CAD build for the part. Positions are in the model's coordinates, mm. A direction names the side the tool comes from. Round coordinates to 2 decimals unless told otherwise and drop trailing zeros. Order: outer loops, then holes, each group sorted by start corner. A loop starts at its lowest first (then second) coordinate and runs counter-clockwise, first axis right, second up.
```python
from build123d import *

# Parameters (mm, degrees)
EXTRUDE_2_DEPTH          = 12.2
SKETCH_5_W               = 3
SKETCH_5_H               = 8.5
CUT_EXTRUDE_1_DEPTH      = 22.5
SKETCH_6_R               = 1.4
EXTRUDE_3_DEPTH          = 2.5
SKETCH_7_W               = 12.2
SKETCH_7_H               = 1
CUT_EXTRUDE_2_DEPTH      = 1
CUT_EXTRUDE_2_DEPTH_BACK = 32.1
EXTRUDE_4_DEPTH          = 0.2
EXTRUDE_5_DEPTH          = 0.2
SKETCH_10_W              = 32.1
SKETCH_10_H              = 20.5
EXTRUDE_6_DEPTH          = 2
SKETCH_11_W              = 32.1
SKETCH_11_H              = 20.5
EXTRUDE_7_DEPTH          = 2


with BuildPart() as part:
    # 草图4 → 凸台-拉伸2 (new body)
    with BuildSketch(Plane.XY):
        Polygon((-11.55, 0), (11.55, 0), (11.55, 17), (16.05, 17), (16.05, -4.5), (-16.05, -4.5), (-16.05, 17), (-11.55, 17), align=None)
    extrude(amount=EXTRUDE_2_DEPTH)

    # 草图5 → 切除-拉伸1 (cut, through all)
    with BuildSketch(Plane.XZ.offset(4.5)):
        with Locations((-10.05, 4.25)):
            Rectangle(SKETCH_5_W, SKETCH_5_H)
    extrude(amount=-CUT_EXTRUDE_1_DEPTH, mode=Mode.SUBTRACT)

    # 草图6 → 凸台-拉伸3 (add)
    with BuildSketch(Plane(origin=(0, 17, 0), x_dir=(1, 0, 0), z_dir=(0, 1, 0))):
        with Locations((13.8, -6.1)):
            Circle(SKETCH_6_R)
        with Locations((-13.8, -6.1)):
            Circle(SKETCH_6_R)
    extrude(amount=EXTRUDE_3_DEPTH)

    # 草图7 → 切除-拉伸2 (cut, two sides)
    with BuildSketch(Plane(origin=(16.05, 0, 0), x_dir=(0, 0, -1), z_dir=(1, 0, 0))) as cut_extrude_2_sk:
        with Locations((-6.1, -4)):
            Rectangle(SKETCH_7_W, SKETCH_7_H)
    extrude(amount=CUT_EXTRUDE_2_DEPTH, mode=Mode.SUBTRACT)
    extrude(cut_extrude_2_sk.sketch, amount=-CUT_EXTRUDE_2_DEPTH_BACK, mode=Mode.SUBTRACT)

    # 草图8 → 凸台-拉伸4 (add)
    with BuildSketch(Plane.XY.offset(12.2)):
        Polygon((-11.55, 17), (-16.05, 17), (-16.05, -3.5), (16.05, -3.5), (16.05, 17), (11.55, 17), (11.55, 0), (-11.55, 0), align=None)
    extrude(amount=EXTRUDE_4_DEPTH)

    # 草图9 → 凸台-拉伸5 (add)
    with BuildSketch(Plane.XY.offset(12.4)):
        Polygon((-11.55, 0), (-11.55, 17), (-16.05, 17), (-16.05, -3.5), (16.05, -3.5), (16.05, 17), (11.55, 17), (11.55, 0), align=None)
    extrude(amount=EXTRUDE_5_DEPTH)

    # 草图10 → 凸台-拉伸6 (add)
    with BuildSketch(Plane.XY.offset(12.6)):
        with Locations((0, 6.75)):
            Rectangle(SKETCH_10_W, SKETCH_10_H)
    extrude(amount=EXTRUDE_6_DEPTH)

    # 草图11 → 凸台-拉伸7 (add)
    with BuildSketch(Plane(origin=(0, 0, 0), x_dir=(-1, 0, 0), z_dir=(0, 0, -1))):
        with Locations((0, 6.75)):
            Rectangle(SKETCH_11_W, SKETCH_11_H)
    extrude(amount=EXTRUDE_7_DEPTH)


solid = part.part
```
1. Drill centre lines: line 1 (X direction, y = -0.75, z = 0.25); line 2 (Z direction, x = -9.5, y = 12); line 3 (X direction, y = 14, z = 2). Where is each one in solid material? Low to high.
2. Cut at B-B, the plane x = -9. Write the cut outline in (y, z).
3. Tool access for faces 5 (the face through (-8.55, -2, 4)), 6 (the face through (11.55, 9, 6)), 7 (the face through (0, 7, -2)): list every direction of +Z, -Z, +X, -X, +Y, -Y with a clear straight run to the whole face (end or side of a thin tool).
4. Mould opens along X. For faces 1 (the face through (14, 19.5, 6)), 2 (the face through (16.05, 7, 6)), 3 (the face through (-16.05, 7, 6)), 4 (the face through (-10, -2, 8.5)) say: released by +X, released by -X, zero draft, split by the parting line, or undercut.
5. Cut at C-C, the plane y = 10.75. Write the cut outline in (x, z), and give its area (3 significant figures).
6. Pin check, flat tips, straight feed: P1, Ø8.5, axis at x = 4.5, z = 4, coming from the +Y side; P2, Ø4, axis at x = 3, z = 4, coming from the +Y side. Stop position of each tip, or through.
7. Cut at A-A, the plane z = 6.1. Write the cut outline in (x, y).
8. Cut at D-D, the plane x = 9. Write the cut outline in (y, z), and give its area (3 significant figures).
Outcome:
1. line 1: x = -16.05 to -11.55, -8.55 to 16.05
1. line 2: z = -2 to 0, 12.6 to 14.6
1. line 3: x = -16.05 to -11.55, 11.55 to 16.05
2. outline: (-3.5, -2) - (17, -2) - (17, 0) - (-3.5, 0) - close; (-3.5, 8.5) - (0, 8.5) - (0, 12.6) - (17, 12.6) - (17, 14.6) - (-3.5, 14.6) - close
3. face 5: +Y, -Y
3. face 6: +Y
3. face 7: -Z, +X, -X, +Y, -Y
4. face 1: zero draft
4. face 2: released by +X
4. face 3: released by -X
4. face 4: undercut
5. outline: (-16.05, -2) - (16.05, -2) - (16.05, 14.6) - (-16.05, 14.6) - close; hole (-11.55, 0) - (11.55, 0) - (11.55, 12.6) - (-11.55, 12.6) - close
5. area: 242 mm2
6. P1: stops at y = 17
6. P2: stops at y = 0
7. outline: (-16.05, -3.5) - (-11.55, -3.5) - (-11.55, 17) - (-12.4, 17) - (-12.4, 19.5) - (-15.2, 19.5) - (-15.2, 17) - (-16.05, 17) - close; (-8.55, -3.5) - (16.05, -3.5) - (16.05, 17) - (15.2, 17) - (15.2, 19.5) - (12.4, 19.5) - (12.4, 17) - (11.55, 17) - (11.55, 0) - (-8.55, 0) - close
8. outline: (-3.5, -2) - (17, -2) - (17, 0) - (0, 0) - (0, 12.6) - (17, 12.6) - (17, 14.6) - (-3.5, 14.6) - close
8. area: 126 mm2
